```python
from build123d import *

# Parameters (mm, degrees)
F1_W     = 38.1
F1_H     = 76.2
F2_DEPTH = 6.35
F0_W     = 609.6
F0_H     = 76.2
F3_DEPTH = 25.4
F4_W     = 31.75
F4_H     = 69.85
F5_DEPTH = 4.318
F6_R     = 6.35
F6_R_2   = 2.413
F7_DEPTH = 12.7


with BuildPart() as f2:
    # F1 (on face) → F2 (new body)
    with BuildSketch(Plane.XY):
        with Locations((31.75, 38.1)):
            Rectangle(F1_W, F1_H)
    extrude(amount=F2_DEPTH)



with BuildPart() as f2b:
    # F1 (on face) → F2, piece 2 (new body)
    with BuildSketch(Plane.XY):
        with Locations((76.708, 38.1)):
            Rectangle(F1_W, F1_H)
    extrude(amount=F2_DEPTH)


with BuildPart() as f2c:
    # F1 (on face) → F2, piece 3 (new body)
    with BuildSketch(Plane.XY):
        with Locations((121.666, 38.1)):
            Rectangle(F1_W, F1_H)
    extrude(amount=F2_DEPTH)


with BuildPart() as f2d:
    # F1 (on face) → F2, piece 4 (new body)
    with BuildSketch(Plane.XY):
        with Locations((166.624, 38.1)):
            Rectangle(F1_W, F1_H)
    extrude(amount=F2_DEPTH)


with BuildPart() as f2e:
    # F1 (on face) → F2, piece 5 (new body)
    with BuildSketch(Plane.XY):
        with Locations((211.582, 38.1)):
            Rectangle(F1_W, F1_H)
    extrude(amount=F2_DEPTH)


with BuildPart() as f2f:
    # F1 (on face) → F2, piece 6 (new body)
    with BuildSketch(Plane.XY):
        with Locations((256.54, 38.1)):
            Rectangle(F1_W, F1_H)
    extrude(amount=F2_DEPTH)


with BuildPart() as f2g:
    # F1 (on face) → F2, piece 7 (new body)
    with BuildSketch(Plane.XY):
        with Locations((301.498, 38.1)):
            Rectangle(F1_W, F1_H)
    extrude(amount=F2_DEPTH)


with BuildPart() as f2h:
    # F1 (on face) → F2, piece 8 (new body)
    with BuildSketch(Plane.XY):
        with Locations((346.456, 38.1)):
            Rectangle(F1_W, F1_H)
    extrude(amount=F2_DEPTH)


with BuildPart() as f2i:
    # F1 (on face) → F2, piece 9 (new body)
    with BuildSketch(Plane.XY):
        with Locations((391.414, 38.1)):
            Rectangle(F1_W, F1_H)
    extrude(amount=F2_DEPTH)


with BuildPart() as f2j:
    # F1 (on face) → F2, piece 10 (new body)
    with BuildSketch(Plane.XY):
        with Locations((436.372, 38.1)):
            Rectangle(F1_W, F1_H)
    extrude(amount=F2_DEPTH)


with BuildPart() as f2k:
    # F1 (on face) → F2, piece 11 (new body)
    with BuildSketch(Plane.XY):
        with Locations((481.33, 38.1)):
            Rectangle(F1_W, F1_H)
    extrude(amount=F2_DEPTH)


with BuildPart() as f2l:
    # F1 (on face) → F2, piece 12 (new body)
    with BuildSketch(Plane.XY):
        with Locations((526.288, 38.1)):
            Rectangle(F1_W, F1_H)
    extrude(amount=F2_DEPTH)


with BuildPart() as f2_1:
    add(f2.part)

    add(f2b.part)  # F3 merges F2b

    add(f2c.part)  # F3 merges F2c

    add(f2d.part)  # F3 merges F2d

    add(f2e.part)  # F3 merges F2e

    add(f2f.part)  # F3 merges F2f

    add(f2g.part)  # F3 merges F2g

    add(f2h.part)  # F3 merges F2h

    add(f2i.part)  # F3 merges F2i

    add(f2j.part)  # F3 merges F2j

    add(f2k.part)  # F3 merges F2k

    add(f2l.part)  # F3 merges F2l
    # F0 (on Top) → F3 (join)
    with BuildSketch(Plane.XY):
        with Locations((304.8, 38.1)):
            Rectangle(F0_W, F0_H)
    extrude(amount=-F3_DEPTH)

    # F4 (on face) → F5 (join)
    with BuildSketch(Plane.XY.offset(6.35)):
        with Locations((31.75, 38.1)):
            Rectangle(F4_W, F4_H)
        with Locations((76.708, 38.1)):
            Rectangle(F4_W, F4_H)
        with Locations((121.666, 38.1)):
            Rectangle(F4_W, F4_H)
        with Locations((166.624, 38.1)):
            Rectangle(F4_W, F4_H)
        with Locations((211.582, 38.1)):
            Rectangle(F4_W, F4_H)
        with Locations((256.54, 38.1)):
            Rectangle(F4_W, F4_H)
        with Locations((301.498, 38.1)):
            Rectangle(F4_W, F4_H)
        with Locations((346.456, 38.1)):
            Rectangle(F4_W, F4_H)
        with Locations((391.414, 38.1)):
            Rectangle(F4_W, F4_H)
        with Locations((436.372, 38.1)):
            Rectangle(F4_W, F4_H)
        with Locations((481.33, 38.1)):
            Rectangle(F4_W, F4_H)
        with Locations((526.288, 38.1)):
            Rectangle(F4_W, F4_H)
    extrude(amount=F5_DEPTH)

    # F6 (on face) → F7 (cut)
    with BuildSketch(Plane.XY.offset(10.668)):
        with Locations((22.479, 66.421)):
            Circle(F6_R)
        with Locations((67.437, 66.421)):
            Circle(F6_R)
        with Locations((112.395, 66.421)):
            Circle(F6_R)
        with Locations((157.353, 66.421)):
            Circle(F6_R)
        with Locations((202.311, 66.421)):
            Circle(F6_R)
        with Locations((247.269, 66.421)):
            Circle(F6_R)
        with Locations((310.769, 66.421)):
            Circle(F6_R)
        with Locations((355.727, 66.421)):
            Circle(F6_R)
        with Locations((400.685, 66.421)):
            Circle(F6_R)
        with Locations((445.643, 66.421)):
            Circle(F6_R)
        with Locations((490.601, 66.421)):
            Circle(F6_R)
        with Locations((535.559, 66.421)):
            Circle(F6_R)
        with Locations((21.8821, 37.4497737813)):
            Circle(F6_R_2)
        with Locations((21.8821, 19.1922262187)):
            Circle(F6_R_2)
        with Locations((37.6936, 28.321)):
            Circle(F6_R_2)
        with Locations((66.8401, 37.4497737813)):
            Circle(F6_R_2)
        with Locations((82.6516, 28.321)):
            Circle(F6_R_2)
        with Locations((66.8401, 19.1922262187)):
            Circle(F6_R_2)
        with Locations((111.7981, 37.4497737813)):
            Circle(F6_R_2)
        with Locations((127.6096, 28.321)):
            Circle(F6_R_2)
        with Locations((111.7981, 19.1922262187)):
            Circle(F6_R_2)
        with Locations((156.7561, 37.4497737813)):
            Circle(F6_R_2)
        with Locations((172.5676, 28.321)):
            Circle(F6_R_2)
        with Locations((156.7561, 19.1922262187)):
            Circle(F6_R_2)
        with Locations((201.7141, 37.4497737813)):
            Circle(F6_R_2)
        with Locations((217.5256, 28.321)):
            Circle(F6_R_2)
        with Locations((201.7141, 19.1922262187)):
            Circle(F6_R_2)
        with Locations((246.6721, 37.4497737813)):
            Circle(F6_R_2)
        with Locations((262.4836, 28.321)):
            Circle(F6_R_2)
        with Locations((246.6721, 19.1922262187)):
            Circle(F6_R_2)
        with Locations((311.3786, 37.465)):
            Circle(F6_R_2)
        with Locations((311.3786, 19.2024)):
            Circle(F6_R_2)
        with Locations((295.5627244608, 28.3337)):
            Circle(F6_R_2)
        with Locations((340.5207244608, 28.3337)):
            Circle(F6_R_2)
        with Locations((356.3366, 19.2024)):
            Circle(F6_R_2)
        with Locations((356.3366, 37.465)):
            Circle(F6_R_2)
        with Locations((385.4787244608, 28.3337)):
            Circle(F6_R_2)
        with Locations((401.2946, 19.2024)):
            Circle(F6_R_2)
        with Locations((401.2946, 37.465)):
            Circle(F6_R_2)
        with Locations((430.4367244608, 28.3337)):
            Circle(F6_R_2)
        with Locations((446.2526, 19.2024)):
            Circle(F6_R_2)
        with Locations((446.2526, 37.465)):
            Circle(F6_R_2)
        with Locations((475.3947244608, 28.3337)):
            Circle(F6_R_2)
        with Locations((491.2106, 19.2024)):
            Circle(F6_R_2)
        with Locations((491.2106, 37.465)):
            Circle(F6_R_2)
        with Locations((520.3527244608, 28.3337)):
            Circle(F6_R_2)
        with Locations((536.1686, 19.2024)):
            Circle(F6_R_2)
        with Locations((536.1686, 37.465)):
            Circle(F6_R_2)
    extrude(amount=-F7_DEPTH, mode=Mode.SUBTRACT)


solid = f2_1.part
```
The listing builds one solid part. Answer for the finished solid, in the listing's coordinates (mm). A direction names the side the tool comes from. Round coordinates to 2 decimals unless told otherwise and drop trailing zeros. Use CSV: the item, a comma, the result in double quotes. Start each with the question number.
(1) Which of the six approach directions +Z, -Z, +X, -X, +Y, -Y give full straight-line access (tool end or side, diameter ignored) to faces 4 (the face through (152.67, 70.71, 4.41)), 5 (the face through (121, 39, 10.668)), 6 (the face through (577, 39, 0))?
(2) Consider L1, parallel to Z at x = 237, y = 38.5; L2, parallel to Y at x = 341.5, z = 7 (3 decimals); L3, parallel to Z at x = 365, y = 11. Determine where each line is inside the solid, lowest interval first. Write a range as from..to.
(3) Each of these flat-tipped pins is pushed along its axis until it touches: pin 1 (2 mm diameter, centred on y = 35.5, z = 9, fed in from -X) (3 decimals); pin 2 (12 mm diameter, centred on x = 91, z = -18.5, fed in from -Y); pin 3 (2 mm diameter, centred on x = 116, z = 9, fed in from +Y) (3 decimals); pin 4 (1.4 mm diameter, centred on x = 384.5, y = 29.5, fed in from +Z). Where does it stop, or does it pass through?
(4) The mould has two halves that part along Y. Classify faces 1 (the face through (439.3, 66.7, 4.4)), 2 (the face through (301, 0, -9)), 3 (the face through (105, 41, 6.35)): released by +Y, released by -Y, zero draft, split by the parting line, or undercut.
A:
1,face 4,"+Z"
1,face 5,"+Z, +X, -X, +Y, -Y"
1,face 6,"+Z, +X, +Y, -Y"
2,L1,"z = -25.4..0"
2,L2,"y = 3.175..26.128, 30.539..73.025"
2,L3,"z = -25.4..6.35"
3,pin 1,"stops at x = 15.875"
3,pin 2,"stops at y = 0"
3,pin 3,"stops at y = 73.025"
3,pin 4,"stops at z = -2.03"
4,face 1,"undercut"
4,face 2,"released by -Y"
4,face 3,"zero draft"
